Autodesk Inventor part; units mm, degrees
ref_plane "YZ Plane" through (0, 0, 0) normal (1, 0, 0) x (0, 1, 0)
ref_plane "XZ Plane" through (0, 0, 0) normal (0, 1, 0) x (-1, 0, 0)
ref_plane "XY Plane" through (0, 0, 0) normal (0, 0, 1) x (1, 0, 0)
sketch "Sketch1" plane through (0, 0, 0) normal (0, 1, 0) x (-1, 0, 0)
  circle A0 centre (0, 0) radius 57.1686
  circle A1 centre (0, 0) radius 33.1656 construction
  circle A2 centre (0, -33.1656) radius 14.2875
  circle A3 centre (31.5424, -10.2487) radius 14.2875
  circle A4 centre (19.4943, 26.8315) radius 14.2875
  circle A5 centre (-19.4943, 26.8315) radius 14.2875
  circle A6 centre (-31.5424, -10.2487) radius 14.2875
  dimension "wheelFilterDiameter" = 66.3312
  dimension "wheelOuterDiameter" = 114.3372
  dimension "filterThreadDiameter" = 28.575
  dimension "d5" = 360
extrude "Extrusion5" add sketch "Sketch1" against normal blind 3.175
sketch "Sketch5" plane through (0, 0, 0) normal (0, 1, 0) x (1, 0, 0)
  arc A0 (35.921, 35.921) -> (0, 50.8) centre (0, 0) ccw construction
  line L0 (0, 50.8) -> (0, -50.8) construction
  line L1 (50.8, 0) -> (-50.8, 0) construction
  line L2 (0, 0) -> (35.921, 35.921) construction
  line L3 (23.0912, 41.7997) -> (25.7305, 46.4819)
  line L4 (25.7305, 46.4819) -> (23.9488, 47.4861)
  line L5 (23.9488, 47.4861) -> (24.303, 48.1144)
  line L6 (24.303, 48.1144) -> (28.572, 45.7081)
  line L7 (28.572, 45.7081) -> (28.2178, 45.0798)
  line L8 (28.2178, 45.0798) -> (26.4362, 46.084)
  line L9 (26.4362, 46.084) -> (23.797, 41.4019)
  line L10 (23.797, 41.4019) -> (23.0912, 41.7997)
  spline S0 degree 2 poles (32.7583, 41.9026) (32.8009, 41.3717) (32.4178, 40.1854) (31.9717, 39.5691) knots 0 0 0 1 2 2 2
  spline S1 degree 2 poles (31.9717, 39.5691) (31.5371, 38.9689) (30.5291, 38.2167) (30.0034, 38.0971) knots 0 0 0 1 2 2 2
  spline S2 degree 2 poles (30.0034, 38.0971) (29.4502, 37.9731) (28.4083, 38.2273) (27.9242, 38.5778) knots 0 0 0 1 2 2 2
  spline S3 degree 2 poles (27.9242, 38.5778) (27.424, 38.9399) (26.8699, 39.8594) (26.8182, 40.403) knots 0 0 0 1 2 2 2
  spline S4 degree 2 poles (26.8182, 40.403) (26.7716, 40.9368) (27.1656, 42.1213) (27.606, 42.7295) knots 0 0 0 1 2 2 2
  spline S5 degree 2 poles (27.606, 42.7295) (28.055, 43.3498) (29.0467, 44.0711) (29.5771, 44.2055) knots 0 0 0 1 2 2 2
  spline S6 degree 2 poles (29.5771, 44.2055) (30.1027, 44.3251) (31.1533, 44.083) (31.6495, 43.7238) knots 0 0 0 1 2 2 2
  spline S7 degree 2 poles (31.6495, 43.7238) (32.1536, 43.3588) (32.707, 42.4215) (32.7583, 41.9026) knots 0 0 0 1 2 2 2
  spline S8 degree 2 poles (31.2874, 40.0645) (31.6408, 40.5527) (31.9762, 41.4625) (31.9637, 41.8496) knots 0 0 0 1 2 2 2
  spline S9 degree 2 poles (31.9637, 41.8496) (31.9531, 42.2477) (31.5862, 42.9035) (31.2421, 43.1527) knots 0 0 0 1 2 2 2
  spline S10 degree 2 poles (31.2421, 43.1527) (30.886, 43.4105) (30.1702, 43.5505) (29.7749, 43.4342) knots 0 0 0 1 2 2 2
  spline S11 degree 2 poles (29.7749, 43.4342) (29.3963, 43.324) (28.6378, 42.7144) (28.2902, 42.2342) knots 0 0 0 1 2 2 2
  spline S12 degree 2 poles (28.2902, 42.2342) (27.5863, 41.2618) (27.6552, 39.6385) (28.3395, 39.1431) knots 0 0 0 1 2 2 2
  spline S13 degree 2 poles (28.3395, 39.1431) (29.0238, 38.6477) (30.5835, 39.0921) (31.2874, 40.0645) knots 0 0 0 1 2 2 2
  spline S14 degree 2 poles (36.5539, 37.0614) (36.2883, 36.7688) (35.6016, 36.4313) (35.2491, 36.4177) knots 0 0 0 1 2 2 2
  spline S15 degree 2 poles (35.2491, 36.4177) (34.8058, 36.3997) (33.9572, 36.7363) (33.4743, 37.1746) knots 0 0 0 1 2 2 2
  line L11 (33.4743, 37.1746) -> (32.9659, 37.6361)
  line L12 (32.9659, 37.6361) -> (31.4386, 35.9534)
  line L13 (31.4386, 35.9534) -> (30.8387, 36.4979)
  line L14 (30.8387, 36.4979) -> (34.9357, 41.0119)
  line L15 (34.9357, 41.0119) -> (36.0697, 39.9826)
  spline S16 degree 2 poles (36.0697, 39.9826) (36.4721, 39.6174) (36.9159, 38.9744) (36.9956, 38.6286) knots 0 0 0 1 2 2 2
  spline S17 degree 2 poles (36.9956, 38.6286) (37.0919, 38.2276) (36.8958, 37.4382) (36.5539, 37.0614) knots 0 0 0 1 2 2 2
  spline S18 degree 2 poles (35.9117, 37.6109) (36.1242, 37.845) (36.2754, 38.3349) (36.2104, 38.594) knots 0 0 0 1 2 2 2
  spline S19 degree 2 poles (36.2104, 38.594) (36.154, 38.8186) (35.8433, 39.2407) (35.5617, 39.4964) knots 0 0 0 1 2 2 2
  line L16 (35.5617, 39.4964) -> (35.0642, 39.9479)
  line L17 (35.0642, 39.9479) -> (33.4307, 38.1482)
  line L18 (33.4307, 38.1482) -> (33.8404, 37.7764)
  spline S20 degree 2 poles (33.8404, 37.7764) (34.2062, 37.4443) (34.7623, 37.153) (35.0481, 37.1739) knots 0 0 0 1 2 2 2
  spline S21 degree 2 poles (35.0481, 37.1739) (35.3063, 37.1864) (35.7159, 37.395) (35.9117, 37.6109) knots 0 0 0 1 2 2 2
  dimension "d25" = 101.6
extrude "Extrusion6" cut sketch "Sketch5" against normal blind 1.016
sketch "Sketch6" plane through (0, 0, 0) normal (0, 1, 0) x (1, 0, 0)
  circle A0 centre (0, 0) radius 6.477
  dimension "d28" = 12.954
extrude "Extrusion7" cut sketch "Sketch6" against normal through all
sketch "Sketch8" plane through (0, -3.175, 0) normal (0, -1, 0) x (1, 0, 0)
  circle A0 centre (0, 0) radius 57.1686
  circle A1 centre (0, 0) radius 54.6286
  dimension "d38" = 114.3372
  dimension "d39" = 2.54
extrude "Extrusion8" add sketch "Sketch8" along normal blind 9.525
sketch "Sketch9" plane through (0, 0, 0) normal (0, 1, 0) x (1, 0, 0)
  circle A0 centre (0, 0) radius 6.477 construction
  circle A1 centre (0, 0) radius 38.1 construction
  line L0 (0, 0) -> (38.1, 0) construction
  line L1 (0, 0) -> (36.2353, -11.7735) construction
  circle A2 centre (19.4943, -26.8315) radius 14.2875 construction
  circle A3 centre (31.5424, 10.2487) radius 14.2875 construction
  line L2 (36.2353, -11.7735) -> (38.0188, -2.4866) construction
  circle A4 centre (31.5424, 10.2487) radius 14.2875 construction
  line L3 (36.2353, -11.7735) -> (32.2194, -20.3352) construction
  point P0 (22.3946, 30.8235)
  point P1 (-22.3946, 30.8235)
  point P2 (-36.2353, -11.7735)
  point P3 (0, -38.1)
  dimension "d42" = 76.2
  dimension "d45" = 360
  dimension "d54" = 18
hole "Hole2" at (36.2353, 0, 11.7735) at (22.3946, 0, -30.8235) at (-22.3946, 0, -30.8235) at (-36.2353, 0, 11.7735) at (0, 0, 38.1) direction (0, -1, 0) diameter 4.4958 end through all
sketch "Sketch11" plane through (0, 0, 0) normal (0, 1, 0) x (1, 0, 0)
  circle A0 centre (0, 0) radius 57.1686
  circle A1 centre (0, 0) radius 47.4531 construction
  point P0 (0, -47.4531)
  point P1 (-45.1306, -14.6638)
  point P2 (-27.8922, 38.3904)
  point P3 (27.8922, 38.3904)
  point P4 (45.1306, -14.6638)
  dimension "d63" = 9.7155
  dimension "d66" = 360
hole "Hole4" at (0, 0, 47.4531) at (-45.1306, 0, 14.6638) at (-27.8922, 0, -38.3904) at (27.8922, 0, -38.3904) at (45.1306, 0, 14.6638) direction (0, -1, 0) diameter 3.81 end through all
equation "\"wheelFilterDiameter\" = 0.318471 * wheelFilterCircumference"
equation "\"wheelOuterDiameter\" = filterDiameter + wheelFilterDiameter + 2 * distanceFromFilterToEdge"
equation "\"d23\" = filterWheelThickness"
equation "\"d26\" = textDepth"
equation "\"d28\" = centerHoleDiameter"
equation "\"distanceBetweenFilters\" = 12.7"
equation "\"distanceFromFilterToEdge\" = 9.525"
equation "\"filterDiameter\" = 28.956"
equation "\"filterWheelThickness\" = 3.175"
equation "\"textDepth\" = 1.016"
equation "\"centerHoleDiameter\" = 12.954"
properties part number "filterHolder" material "PBT Plastic"
Geometry: final body of the model. Coordinates: model frame, mm. A direction names the side the tool comes from. Give positions to 0.01 mm unless a question says otherwise; leave off trailing zeros. Loops run counter-clockwise (first coordinate to the right, second up) from the corner with the lowest first, then second, coordinate; pieces in that order, holes last. Notation, with made-up numbers: (23.5, 75) - (71.5, 75) arc R21 cw to (71.5, 80) - close; hole circle Ø9 at (1.25, 29.5). An arc over 180 degrees is marked (long way). One line per question, with ' | ' between items. Start each with the question number.
(1) Contact query for flat-ended pins moving along their axis: pin 1 (3 mm diameter, centred on y = -9, z = 17.5, fed in from -X); pin 2 (12 mm diameter, centred on x = -28.5, z = 8.5, fed in from -Y) (3 decimals); pin 3 (2 mm diameter, centred on y = -8, z = -41.5, fed in from +X). Output: stop coordinate, or through.
(2) Section query A-A on x = 0. Return loops of the section in (y, z) (3 decimals).
(3) Section query B-B on z = 38.1. Return loops of the section in (x, y) (3 decimals).
(4) Section query D-D on y = -4.75. Return loops of the section in (x, z), then the cut area to 3 significant figures.
(5) Section query C-C on z = -16. Return loops of the section in (x, y) (3 decimals).
(6) Ray query, line 1 (Z direction, x = 0, y = -0.65); line 2 (X direction, y = -10.25, z = 0.5); line 3 (X direction, y = -2.25, z = 27). Return the intervals inside material, ascending. Write a range as from..to.
(7) Reachability of faces 1 (the flat face through (35, 0, -38)), 2 (the cylindrical face through (-54.576, -7.871, -2.402)), 3 (the flat face through (34, -1.016, -37)) from +Z, -Z, +X, -X, +Y, -Y: full face, straight path, thin tool, end or side. Return the list, or none.
(8) Pull-direction query (Z, two-part tool) for faces 4 (the flat face through (46.3, -12.7, -29.4)), 5 (the cylindrical face through (-46.737, -1.61, 15.688)); classes: released by +Z, released by -Z, zero draft, split by the parting line, or undercut.
The answers:
1) pin 1: x = -54.88 | pin 2: y = -3.175 | pin 3: x = 40.35
2) outline: (-12.7, -57.169) - (0, -57.169) - (0, -47.453) - (-3.175, -47.453) - (-3.175, -54.629) - (-12.7, -54.629) - close; (-12.7, 54.629) - (-3.175, 54.629) - (-3.175, 49.358) - (0, 49.358) - (0, 57.169) - (-12.7, 57.169) - close; (-3.175, -18.878) - (0, -18.878) - (0, -6.477) - (-3.175, -6.477) - close; (-3.175, 6.477) - (0, 6.477) - (0, 35.852) - (-3.175, 35.852) - close; (-3.175, 40.348) - (0, 40.348) - (0, 45.548) - (-3.175, 45.548) - close
3) outline: (-42.622, -12.7) - (-39.149, -12.7) - (-39.149, -3.175) - (-28.278, -3.175) - (-28.278, 0) - (-42.622, 0) - close; (-10.711, -3.175) - (-2.248, -3.175) - (-2.248, 0) - (-10.711, 0) - close; (2.248, -3.175) - (10.711, -3.175) - (10.711, 0) - (2.248, 0) - close; (28.278, -3.175) - (39.149, -3.175) - (39.149, -12.7) - (42.622, -12.7) - (42.622, 0) - (28.278, 0) - close
4) outline: circle Ø114.34 at (0, 0); hole circle Ø109.26 at (0, 0) | area: 892 mm2
5) outline: (-54.884, -12.7) - (-52.233, -12.7) - (-52.233, -3.175) - (-44.621, -3.175) - (-44.621, 0) - (-54.884, 0) - close; (-18.464, -3.175) - (18.464, -3.175) - (18.464, 0) - (-18.464, 0) - close; (44.621, -3.175) - (52.233, -3.175) - (52.233, -12.7) - (54.884, -12.7) - (54.884, 0) - (44.621, 0) - close
6) line 1: -57.17..-47.45, -18.88..-6.48, 6.48..35.85, 40.35..45.55, 49.36..57.17 | line 2: -57.17..-54.63, 54.63..57.17 | line 3: -50.39..-33.78, -5.21..5.21, 33.78..50.39
7) face 1: +Z, -Z, +X, -X, +Y | face 2: -Y | face 3: +Y
8) face 4: zero draft | face 5: undercut
